Autodesk Inventor part; units mm, degrees
ref_plane "YZ Plane" through (0, 0, 0) normal (1, 0, 0) x (0, 1, 0)
ref_plane "XZ Plane" through (0, 0, 0) normal (0, 1, 0) x (-1, 0, 0)
ref_plane "XY Plane" through (0, 0, 0) normal (0, 0, 1) x (1, 0, 0)
sketch "Sketch1" plane through (0, 0, 0) normal (1, 0, 0) x (0, 1, 0)
  line L0 (0, 0) -> (1.5, 2)
  line L1 (1.5, 2) -> (1.5, 43)
  line L2 (0, 59) -> (0, 0)
  line L3 (11.5, 51) -> (16.5, 51)
  line L4 (16.5, 51) -> (16.5, 101)
  line L5 (16.5, 101) -> (11.5, 101)
  line L6 (1.5, 105) -> (1.5, 120)
  line L7 (1.5, 120) -> (0, 120)
  line L8 (0, 120) -> (0, 59)
  line L9 (0, -24) -> (0, 144)
  line L10 (16.5, 76) -> (-5.6648, 76)
  line L11 (-30.7978, 0) -> (145.133, 0)
  line L12 (11.5, 101) -> (11.5, 105)
  line L13 (11.5, 105) -> (1.5, 105)
  line L14 (11.5, 51) -> (11.5, 47)
  line L15 (11.5, 47) -> (5.5, 47)
  line L16 (5.5, 47) -> (5.5, 43)
  line L17 (5.5, 43) -> (1.5, 43)
  line L18 (0, 0) -> (2, 1.5)
  line L19 (2, 1.5) -> (43, 1.5)
  line L20 (43, 1.5) -> (43, 5.5)
  line L21 (43, 5.5) -> (47, 5.5)
  line L22 (47, 5.5) -> (47, 11.5)
  line L23 (47, 11.5) -> (51, 11.5)
  line L24 (51, 11.5) -> (51, 15)
  line L25 (51, 15) -> (101, 15)
  line L26 (101, 15) -> (101, 11.5)
  line L27 (101, 11.5) -> (112, 11.5)
  line L28 (112, 11.5) -> (112, 1.5)
  line L29 (112, 1.5) -> (120, 1.5)
  line L30 (120, 1.5) -> (120, 0)
  line L31 (-30.7978, 0) -> (145.133, 0)
  line L32 (76, 15) -> (76, 0)
  line L33 (0, 0) -> (120, 0)
  dimension "d0" = 2
  dimension "d3" = 76
  dimension "d4" = 120
  dimension "d5" = 50
  dimension "d7" = 1.5
  dimension "d8" = 10
  dimension "d9" = 4
  dimension "d10" = 4
  dimension "d11" = 4
  dimension "d12" = 6
  dimension "d13" = 4
  dimension "d21" = 2
  dimension "d22" = 1.5
  dimension "d23" = 76
  dimension "d24" = 120
  dimension "d25" = 1.5
  dimension "d26" = 4
  dimension "d27" = 4
  dimension "d28" = 6
  dimension "d29" = 4
  dimension "d30" = 10
  dimension "d31" = 8
  dimension "d32" = 50
  dimension "d33" = 15
  dimension "d42" = 3
revolve "Revolution1" add sketch "Sketch1" angle 360 about axis through (0, -10, 0) along (0, 1, 0) contours L18 L19 L20 L21 L22 L23 L24 L25 L32 L11 | L32 L25 L26 L27 L28 L29 L30 L11
ref_plane "Work Plane2" through (0, 76, 0) normal (0, 1, 0) x (1, 0, 0)
sketch "Sketch4" plane through (0, 76, 0) normal (0, 1, 0) x (1, 0, 0)
  arc A0 (-20, 0) -> (20, 0) centre (0, 0) ccw
  line L0 (-20, 0) -> (-20, 20)
  line L1 (-20, 20) -> (20, 20)
  line L2 (20, 20) -> (20, 0)
  dimension "d35" = 20
  dimension "d36" = 20
extrude "Extrusion3" add sketch "Sketch4" along normal mid plane 10
sketch "Sketch5" plane through (20, 81, -20) normal (0, 0, -1) x (-1, 0, 0)
  line L0 (0, 0) -> (0, -10)
  line L1 (0, -5) -> (40, -5) construction
  line L2 (40, -10) -> (40, 0)
  circle A0 centre (20, -5) radius 25
  point P0 (20, -81)
  dimension "d39" = 50
extrude "Extrusion4" add sketch "Sketch5" along normal blind 8.75
properties part number "spindle"
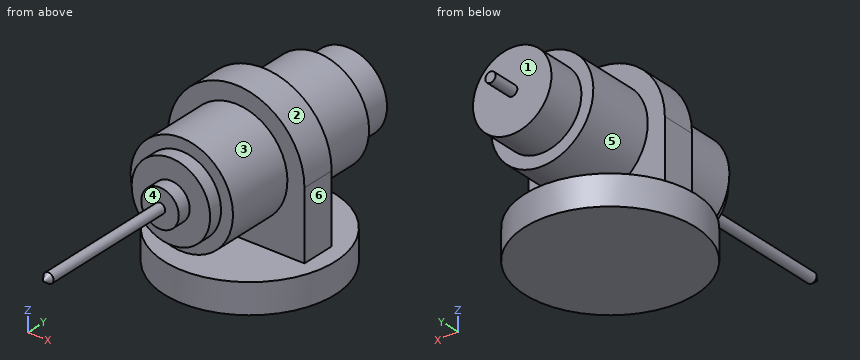
Model file for the job. Use its own axes, mm. Face numbers are marked on the shaded views. A direction names the side the tool comes from. Give positions to 0.01 mm unless a question says otherwise; leave off trailing zeros. Write each loop counter-clockwise with the first axis right and the second up, starting at its lowest first coordinate (ties: lowest second). Pieces come first, ordered by that corner, then holes. Notation, with made-up numbers: (27, 24) - (75, 24) arc R23 cw to (75, 36) - close; hole circle Ø6 at (17.5, -21). An arc over 180 degrees is marked (long way). One line per question, with ' | ' between items. Start each with the question number.
(1) Two-plate mould, pull along Z, no slides. Class the marked faces 1, 2 and 3: +Z half, -Z half, draft (parallel to the pull), parting line (faces both ways), or undercut.
(2) Slice it at A-A on y = 76. Write the cut outline in (x, z), plus the area to 3 significant figures.
(3) Pin check, flat tips, straight feed: P1, Ø12, axis at x = -9.5, z = 12.5, coming from the +Y side; P2, Ø2, axis at x = 13.5, z = -4, coming from the +Y side; P3, Ø3, axis at y = 74, z = -13.5, coming from the -X side. Stop position of each tip, or through.
(4) Slice it at D-D on y = 94. Write the cut outline in (x, z).
(5) 3-axis set-ups, long thin cutter, end or side, ignore diameter. For the marked faces 4, 5 and 6: which of +Z, -Z, +X, -X, +Y, -Y reach the whole face in a straight line?
(6) Slice it at B-B on x = 17.5. Write the cut outline in (y, z).
(7) Wall check: line 1 along Y through (x, z) = (1, -3.5); line 2 along Y through (x, z) = (-15, 7.5); line 3 along X through (y, z) = (75, -21). Give the ranges that are in metal, low to high. Write a range as from..to.
(8) Slice it at C-C on y = 63.5. Write the cut outline in (x, z), plus the area to 3 significant figures.
Results below:
1) face 1: draft | face 2: +Z half | face 3: undercut
2) outline: (-25, -28.75) - (25, -28.75) - (25, -20) - (20, -20) - (20, 0) arc R20 ccw to (-20, 0) - (-20, -20) - (-25, -20) - close | area: 1,870 mm^2
3) P1: y = 112 | P2: y = 101 | P3: x = -20
4) outline: (-17.35, -28.75) - (17.35, -28.75) - (17.35, -20) - (-17.35, -20) - close; circle Ø30 at (0, 0)
5) face 4: -Y | face 5: +Y | face 6: +Z, +X, +Y, -Y
6) outline: (58.15, -28.75) - (93.85, -28.75) - (93.85, -20) - (81, -20) - (81, 9.68) - (71, 9.68) - (71, -20) - (58.15, -20) - close
7) line 1: 43..112 | line 2: 71..81 | line 3: -24.98..24.98
8) outline: (-21.65, -28.75) - (21.65, -28.75) - (21.65, -20) - (-21.65, -20) - close; circle Ø30 at (0, 0) | area: 1,090 mm^2
